```python
from build123d import *

# Parameters (mm, degrees)
EXTRUSION1_DEPTH = 15
ESQUISSE3_R      = 2
EXTRUSION3_DEPTH = 31.646855226
ESQUISSE4_R      = 1.5
EXTRUSION4_DEPTH = 10


with BuildPart() as part:
    # Esquisse1 → Extrusion1 (new body)
    with BuildSketch(Plane.XY):
        Polygon((-1.5, 17.726526316), (-1.5, -2.273473684), (18.5, -2.273473684), (18.5, 17.726526316), (17, 17.726526316), (17, -0.773473684), (0, -0.773473684), (0, 17.726526316), align=None)
    extrude(amount=EXTRUSION1_DEPTH)

    # Esquisse3 → Extrusion3 (cut, through all)
    with BuildSketch(Plane(origin=(18.5, 0, 0), x_dir=(0, 0, -1), z_dir=(1, 0, 0))):
        with Locations(Location((-7.5, 11.726526316, 0), (0, 0, 90))):
            Circle(ESQUISSE3_R)
    extrude(amount=-EXTRUSION3_DEPTH, mode=Mode.SUBTRACT)

    # Esquisse4 → Extrusion4 (cut)
    with BuildSketch(Plane(origin=(0, -0.773473684, 0), x_dir=(1, 0, 0), z_dir=(0, 1, 0))):
        with Locations(Location((3.5, -7.5, 0), (0, 0, 180))):
            Circle(ESQUISSE4_R)
        with Locations(Location((13.5, -7.5, 0), (0, 0, 180))):
            Circle(ESQUISSE4_R)
    extrude(amount=-EXTRUSION4_DEPTH, mode=Mode.SUBTRACT)


solid = part.part
```
Here's how the part is built. I have some questions about the finished solid (model axes, mm). A direction names the side the tool comes from. Coordinates: 2 decimals unless noted, no trailing zeros. Order: outer loops, then holes, each group sorted by start corner. A loop starts at its lowest first (then second) coordinate and runs counter-clockwise, first axis right, second up.
Item 1: I need wall thicknesses on probe 1 along X at (y, z) = (14.5, 10.25); probe 2 along Z at (x, y) = (3.5, -1.5); probe 3 along Y at (x, z) = (8.25, 10). Which ranges of each line are inside material? Lowest first, please.
Response values:
probe 1: x = -1.5 to 0, 17 to 18.5
probe 2: z = 0 to 6, 9 to 15
probe 3: y = -2.27 to -0.77
Item 2: If we section it at C-C, the plane y = 3: List the corners of the cut face in (x, z) for me, then the cut area to 3 significant figures.
Response values:
outline: (-1.5, 0) - (0, 0) - (0, 15) - (-1.5, 15) - close; (17, 0) - (18.5, 0) - (18.5, 15) - (17, 15) - close
area: 45.0 mm2
Item 3: If we section it at B-B, the plane z = 7.5: List the corners of the cut face in (x, y) for me.
Response values:
outline: (-1.5, -2.27) - (2, -2.27) - (2, -0.77) - (0, -0.77) - (0, 9.73) - (-1.5, 9.73) - close; (-1.5, 13.73) - (0, 13.73) - (0, 17.73) - (-1.5, 17.73) - close; (5, -2.27) - (12, -2.27) - (12, -0.77) - (5, -0.77) - close; (15, -2.27) - (18.5, -2.27) - (18.5, 9.73) - (17, 9.73) - (17, -0.77) - (15, -0.77) - close; (17, 13.73) - (18.5, 13.73) - (18.5, 17.73) - (17, 17.73) - close
Item 4: If we section it at D-D, the plane z = 11.75: List the corners of the cut face in (x, y) for me, then the cut area to 3 significant figures.
Response values:
outline: (-1.5, -2.27) - (18.5, -2.27) - (18.5, 17.73) - (17, 17.73) - (17, -0.77) - (0, -0.77) - (0, 17.73) - (-1.5, 17.73) - close
area: 85.5 mm2
Item 5: I'm going to push flat-ended pins straight in: pin 1 Ø1.5 at (x, z) = (15, 11) entering from +Y; pin 2 Ø6 at (x, y) = (5.5, 15.5) entering from -Z. Where does each tip first touch, or does it pass through?
Response values:
pin 1: stops at y = -0.77
pin 2: passes through
Item 6: Which directions (+Z, -Z, +X, -X, +Y, -Y) give clear straight access to the entire face, cutting with the end or side of a thin tool? Please do faces 5 (the face through (17, 9, 7)), 6 (the face through (-1.5, 8, 7)).
Response values:
face 5: +Z, -Z, +Y
face 6: +Z, -Z, -X, +Y, -Y
Item 7: If we section it at A-A, the plane x = 13.5: List the corners of the cut face in (y, z) for me.
Response values:
outline: (-2.27, 0) - (-0.77, 0) - (-0.77, 6) - (-2.27, 6) - close; (-2.27, 9) - (-0.77, 9) - (-0.77, 15) - (-2.27, 15) - close
Item 8: Thinking about a two-plate mould opening in Y: for faces 1 (the face through (8, -1, 0)), 2 (the face through (17.76, 12.802, 9.186)), 3 (the face through (-1, 17.727, 7)), 4 (the face through (-0.739, 12.802, 9.186)), which applies, pulls with the +Y half, pulls with the -Y half, needs draft (parallel to the pull), parting line crosses it, or undercut?
Response values:
face 1: needs draft
face 2: undercut
face 3: pulls with the +Y half
face 4: undercut
